from build123d import *

# Parameters (mm, degrees)
SKETCH1_R           = 21
SKETCH1_R_2         = 8.75
BOSS_EXTRUDE1_DEPTH = 5
SKETCH2_R           = 2.1
SKETCH2_R_2         = 1.6
CUT_EXTRUDE1_DEPTH  = 5
SKETCH3_R           = 17.5
SKETCH3_R_2         = 8.75
BOSS_EXTRUDE2_DEPTH = 35


with BuildPart() as part:
    # Sketch1 → Boss-Extrude1 (new body)
    with BuildSketch(Plane(origin=(0, 0, 0), x_dir=(1, 0, 0), z_dir=(0, 1, 0))):
        Circle(SKETCH1_R)
        Circle(SKETCH1_R_2, mode=Mode.SUBTRACT)
    extrude(amount=BOSS_EXTRUDE1_DEPTH)

    # Sketch2 → Cut-Extrude1 (cut)
    with BuildSketch(Plane.XZ):
        with Locations((-10.253048327, 10.253048327)):
            Circle(SKETCH2_R)
        with Locations((10.253048327, -10.253048327)):
            Circle(SKETCH2_R)
        with Locations((-15, 0)):
            Circle(SKETCH2_R_2)
        with Locations((7.5, 12.990381057)):
            Circle(SKETCH2_R_2)
        with Locations((7.5, -12.990381057)):
            Circle(SKETCH2_R_2)
        with Locations((8.838834765, 8.838834765)):
            Circle(SKETCH2_R_2)
        with Locations((-8.838834765, -8.838834765)):
            Circle(SKETCH2_R_2)
    extrude(amount=-CUT_EXTRUDE1_DEPTH, mode=Mode.SUBTRACT)

    # Sketch3 → Boss-Extrude2 (add)
    with BuildSketch(Plane(origin=(0, 5, 0), x_dir=(1, 0, 0), z_dir=(0, 1, 0))):
        Circle(SKETCH3_R)
        Circle(SKETCH3_R_2, mode=Mode.SUBTRACT)
    extrude(amount=BOSS_EXTRUDE2_DEPTH)


solid = part.part
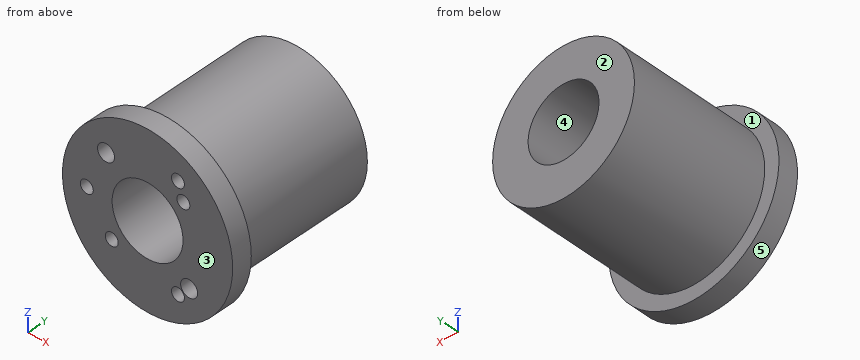
Check sheet for the modelled part. Datum: model origin and axes. Units: mm. Face numbers are marked on the shaded views. A direction names the side the tool comes from. Give positions to 0.01 mm unless a question says otherwise; leave off trailing zeros. Write each loop counter-clockwise with the first axis right and the second up, starting at its lowest first coordinate (ties: lowest second). Pieces come first, ordered by that corner, then holes. Notation, with made-up numbers: M 23.5,68 L 32.5,68 A6 cw 32.5,77 Z; hole C -37,31.5 d8. An arc over 180 degrees is marked long. Use one line per item in the form item = value.
(1) Material ranges on line 1 along Z through (x, y) = (7.5, 3); line 2 along Y through (x, z) = (-17, 5.5); line 3 along Z through (x, y) = (-1.5, 24), recorded low to high.
Answer block:
line_1 = -19.62 to -14.59, -11.39 to -4.51, 4.51 to 7.96, 9.71 to 11.39, 14.59 to 19.62
line_2 = 0 to 5
line_3 = -17.44 to -8.62, 8.62 to 17.44
(2) Section check D-D on x = 3. Record the boundary of the cut face in (y, z).
Answer block:
outline = M 0,-20.78 L 5,-20.78 L 5,-17.24 L 40,-17.24 L 40,-8.22 L 0,-8.22 Z; M 0,8.22 L 40,8.22 L 40,17.24 L 5,17.24 L 5,20.78 L 0,20.78 Z
(3) Draft check along X on the marked faces 3, 4 and 5. Enter one of: pulls with the +X half, pulls with the -X half, needs draft (parallel to the pull), parting line crosses it, or undercut.
Answer block:
face_3 = needs draft
face_4 = undercut
face_5 = parting line crosses it
(4) Section check B-B on x = -5. Record the boundary of the cut face in (y, z), plus the area to 3 significant figures.
Answer block:
outline = M 0,-20.4 L 5,-20.4 L 5,-16.77 L 40,-16.77 L 40,-7.18 L 0,-7.18 Z; M 0,7.18 L 40,7.18 L 40,16.77 L 5,16.77 L 5,20.4 L 0,20.4 Z
area = 803 mm2
(5) Depth check by flat-ended pin: P1, Ø3, axis at y = 35.5, z = -10.5, coming from the -X side; P2, Ø2.5, axis at x = -8.84, z = -8.84, coming from the -Y side; P3, Ø10, axis at y = 22.5, z = 0, coming from the +X side. Enter the tip coordinate at first touch or a pass-through.
Answer block:
P1 = -15.01
P2 = 5
P3 = 17.5
(6) Section check A-A on z = 0. Record the boundary of the cut face in (x, y), plus the area to 3 significant figures.
Answer block:
outline = M -21,0 L -16.6,0 L -16.6,5 L -13.4,5 L -13.4,0 L -8.75,0 L -8.75,40 L -17.5,40 L -17.5,5 L -21,5 Z; M 8.75,0 L 21,0 L 21,5 L 17.5,5 L 17.5,40 L 8.75,40 Z
area = 719 mm2
(7) Section check C-C on y = 22.5. Record the boundary of the cut face in (x, z), plus the area to 3 significant figures.
Answer block:
outline = C 0,0 d35; hole C 0,0 d17.5
area = 722 mm2
(8) Tool access check on the marked faces 1 and 2. Record the directions out of +Z, -Z, +X, -X, +Y, -Y that give a thin tool (end or side, any length) a straight path to the whole face; none if there is none.
Answer block:
face_1 = +Y
face_2 = +Z, -Z, +X, -X, +Y
